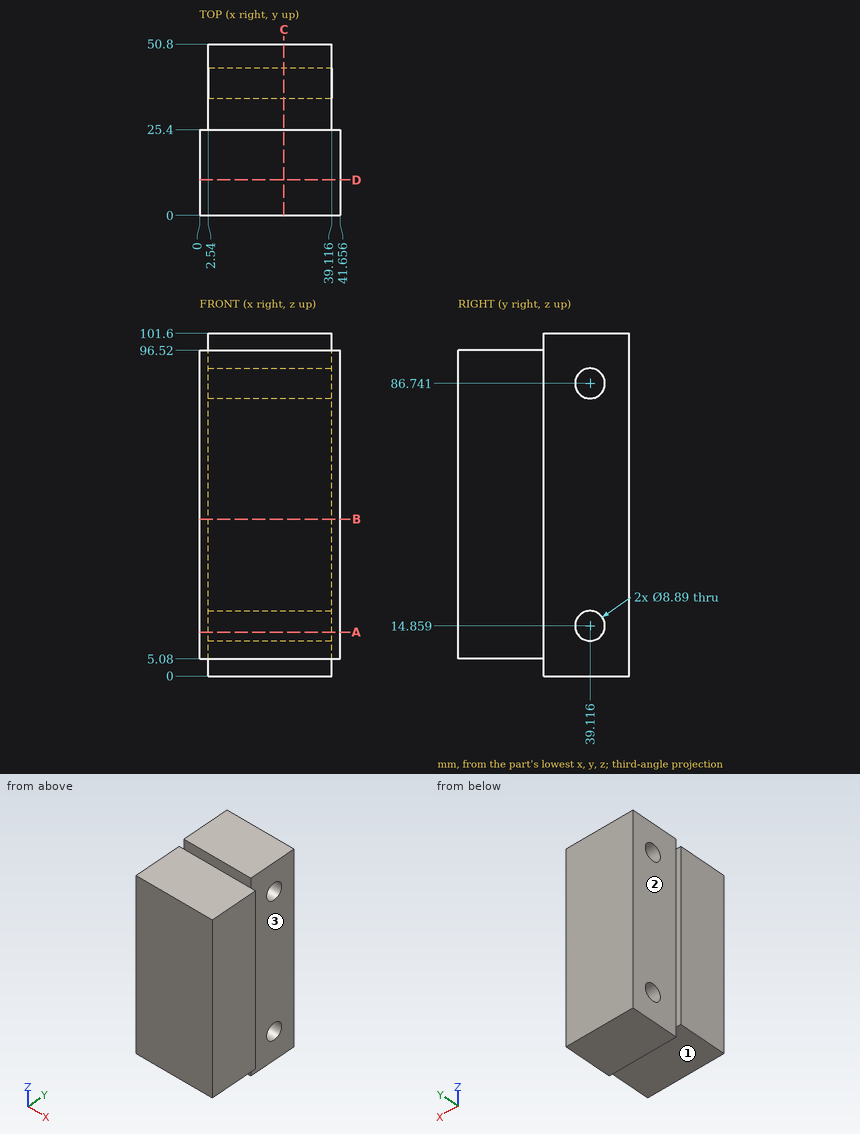
The drawing under review shows one solid part. Ordinate dimensions are in mm from its lowest x, y, z. A direction names the side the tool comes from. Give positions to 0.01 mm unless a question says otherwise; leave off trailing zeros. Order: outer loops, then holes, each group sorted by start corner. A loop starts at its lowest first (then second) coordinate and runs counter-clockwise, first axis right, second up. Notation, with made-up numbers: M -19.75,-21.75 L 25.25,-21.75 A17 ccw 25.25,1.25 Z; hole C -39.5,88 d7. An arc over 180 degrees is marked long. Answer in a Markdown table with one row per item. Add a question column.
1. For pin 1 Ø4 at (y, z) = (42, 32) entering from +X; pin 2 Ø5.5 at (x, z) = (29.5, 2) entering from -Y; pin 3 Ø20.5 at (x, y) = (11.5, 6.5) entering from +Z; pin 4 Ø8 at (y, z) = (39.116, 14.859) entering from +X, all flat-tipped, find the tip position at first contact; note any pin that passes through.
2. Add section C-C on x = 25. State the section outline as (y, z) points (3 decimals), plus the area to 3 significant figures.
3. Add section D-D on y = 10.5. State the section outline as (x, z) points, plus the area to 3 significant figures.
4. Machinability: for the marked faces 1, 2 and 3, which of the approach directions +Z, -Z, +X, -X, +Y, -Y give a long, thin tool a straight path to every point of the face, cutting with its end or side? Answer none if there is none.
5. To check wall thickness, follow line 1 along Z through (x, y) = (21.5, 42); line 2 along Z through (x, y) = (33, 41.5); line 3 along Z through (x, y) = (20.5, 24). State the ranges of each line that lie inside material, in increasing order.
6. Add section A-A on z = 13. State the section outline as (x, y) points.
7. Add section B-B on z = 46.5. State the section outline as (x, y) points.
The answers:
| question | item | result |
|---|---|---|
| 1 | pin 1 | x = 39.12 |
| 1 | pin 2 | y = 25.4 |
| 1 | pin 3 | z = 96.52 |
| 1 | pin 4 | through |
| 2 | outline | M 0,5.08 L 25.4,5.08 L 25.4,0 L 50.8,0 L 50.8,101.6 L 25.4,101.6 L 25.4,96.52 L 0,96.52 Z; hole C 39.116,14.859 d8.89; hole C 39.116,86.741 d8.89 |
| 2 | area | 4,780 mm2 |
| 3 | outline | M 0,5.08 L 41.66,5.08 L 41.66,96.52 L 0,96.52 Z |
| 3 | area | 3,810 mm2 |
| 4 | face 1 | -Z, +X, -X, -Y |
| 4 | face 2 | +Z, -Z, -X, +Y |
| 4 | face 3 | +Z, -Z, +X, +Y |
| 5 | line 1 | 0 to 11.48, 18.24 to 83.36, 90.12 to 101.6 |
| 5 | line 2 | 0 to 11.11, 18.61 to 82.99, 90.49 to 101.6 |
| 5 | line 3 | 5.08 to 96.52 |
| 6 | outline | M 0,0 L 41.66,0 L 41.66,25.4 L 39.12,25.4 L 39.12,35.08 L 2.54,35.08 L 2.54,25.4 L 0,25.4 Z; M 2.54,43.15 L 39.12,43.15 L 39.12,50.8 L 2.54,50.8 Z |
| 7 | outline | M 0,0 L 41.66,0 L 41.66,25.4 L 39.12,25.4 L 39.12,50.8 L 2.54,50.8 L 2.54,25.4 L 0,25.4 Z |
